Check sheet for the modelled part. Datum: model origin and axes. Units: mm. A direction names the side the tool comes from. Give positions to 0.01 mm unless a question says otherwise; leave off trailing zeros. Order: outer loops, then holes, each group sorted by start corner. A loop starts at its lowest first (then second) coordinate and runs counter-clockwise, first axis right, second up. Notation, with made-up numbers: (45.5, -17.75) - (79.5, -17.75) arc R19 cw to (79.5, 2.25) - close; hole circle Ø1 at (84.5, -5). An arc over 180 degrees is marked (long way). Answer in a Markdown table with one row per item.
from build123d import *

# Parameters (mm, degrees)
SKETCH2_W          = 469.9
SKETCH2_H          = 63.5
EXTRUDE1_DEPTH     = 17.78
SKETCH3_W          = 17.78
SKETCH3_H          = 63.5
CUT_EXTRUDE1_DEPTH = 5.08
SKETCH4_R          = 1.5875
CUT_EXTRUDE2_DEPTH = 17.78
SKETCH5_R          = 1.5875
CUT_EXTRUDE3_DEPTH = 17.78


with BuildPart() as part:
    # Sketch2 → Extrude1 (new body)
    with BuildSketch(Plane.XY):
        with Locations((11073.341666666, -5688.0125)):
            Rectangle(SKETCH2_W, SKETCH2_H)
    extrude(amount=-EXTRUDE1_DEPTH)

    # Sketch3 → Cut-Extrude1 (cut)
    with BuildSketch(Plane.XY):
        with Locations((11299.401666666, -5688.0125)):
            Rectangle(SKETCH3_W, SKETCH3_H)
        with Locations((10847.281666666, -5688.0125)):
            Rectangle(SKETCH3_W, SKETCH3_H)
    extrude(amount=-CUT_EXTRUDE1_DEPTH, mode=Mode.SUBTRACT)

    # Sketch4 → Cut-Extrude2 (cut)
    with BuildSketch(Plane.XY):
        with Locations((10847.281666666, -5668.9625)):
            Circle(SKETCH4_R)
        with Locations((10847.281666666, -5707.0625)):
            Circle(SKETCH4_R)
        with Locations((11299.401666666, -5707.0625)):
            Circle(SKETCH4_R)
        with Locations((11299.401666666, -5668.9625)):
            Circle(SKETCH4_R)
    extrude(amount=-CUT_EXTRUDE2_DEPTH, mode=Mode.SUBTRACT)

    # Sketch5 → Cut-Extrude3 (cut)
    with BuildSketch(Plane(origin=(0, 0, -17.78), x_dir=(-1, 0, 0), z_dir=(0, 0, -1))):
        with Locations((-10876.491666666, -5690.78745)):
            Circle(SKETCH5_R)
        with Locations((-10927.291666666, -5690.78745)):
            Circle(SKETCH5_R)
        with Locations((-11219.391666666, -5690.78745)):
            Circle(SKETCH5_R)
        with Locations((-11270.191666666, -5690.78745)):
            Circle(SKETCH5_R)
    extrude(amount=-CUT_EXTRUDE3_DEPTH, mode=Mode.SUBTRACT)


solid = part.part
(1) Access from +Z, -Z, +X, -X, +Y, -Y to the whole of each face (thin tool, end or side, straight path). Record for faces 1 (the flat face through (11299, -5688, -5.08)), 2 (the flat face through (10847, -5688, -5.08)), 3 (the flat face through (11070, -5688, 0)).
Geometry says:
| item | result |
|---|---|
| face 1 | +Z, +X, +Y, -Y |
| face 2 | +Z, -X, +Y, -Y |
| face 3 | +Z, +X, -X, +Y, -Y |
(2) Gauge pin test, flat ends, axial feed: P1, Ø5.5, axis at x = 10849, y = -5692.5, coming from the +Z side; P2, Ø1.5, axis at x = 11249, y = -5692, coming from the +Z side; P3, Ø1.5, axis at y = -5688.5, z = -2, coming from the +X side; P4, Ø1.5, axis at y = -5689.5, z = -3, coming from the -X side. Record the tip position at first contact, or that the pin passes through.
Geometry says:
| item | result |
|---|---|
| P1 | z = -5.08 |
| P2 | z = 0 |
| P3 | x = 11290.51 |
| P4 | x = 10856.17 |
(3) Thickness scan on L1, parallel to X at y = -5706, z = -5.25; L2, parallel to X at y = -5708, z = -13.5; L3, parallel to X at y = -5691.5, z = -16.5. Record the ranges inside material, lowest first.
Geometry says:
| item | result |
|---|---|
| L1 | 10838.39 to 10846.1, 10848.46 to 11298.22, 11300.58 to 11308.29 |
| L2 | 10838.39 to 10846, 10848.56 to 11298.12, 11300.68 to 11308.29 |
| L3 | 10838.39 to 10875.07, 10877.91 to 10925.87, 10928.71 to 11217.97, 11220.81 to 11268.77, 11271.61 to 11308.29 |
(4) Cross-section at A-A, the plane y = -5684.5. Record the cut outline in (x, z).
Geometry says:
| item | result |
|---|---|
| outline | (10838.39, -17.78) - (11308.29, -17.78) - (11308.29, -5.08) - (11290.51, -5.08) - (11290.51, 0) - (10856.17, 0) - (10856.17, -5.08) - (10838.39, -5.08) - close |
